Could you check a few things on this model? Use its own coordinates, in mm. Face numbers are marked on the shaded views. A direction names the side the tool comes from. Round coordinates to 2 decimals unless told otherwise and drop trailing zeros. Loops run counter-clockwise (first coordinate to the right, second up) from the corner with the lowest first, then second, coordinate; pieces in that order, holes last. Notation, with made-up numbers: (-35.75, 63) - (-25.75, 63) arc R20 ccw to (-25.75, 74) - close; hole circle Ø10 at (7.5, 15.25). An arc over 180 degrees is marked (long way). Use one line per item in the form item = value.
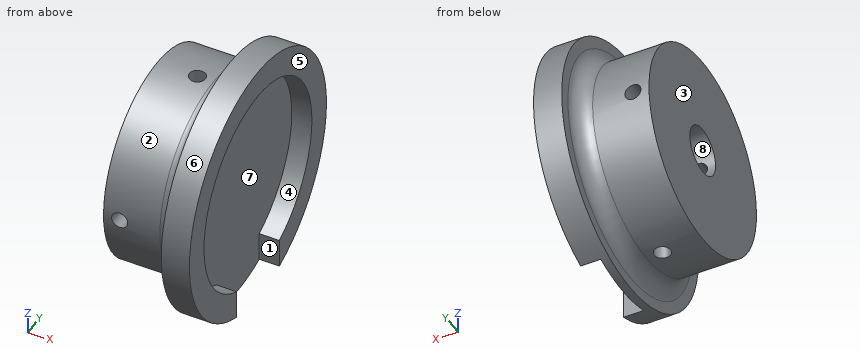
```python
from build123d import *

# Parameters (mm, degrees)
SKETCH_1_R                      = 12.55
EXTRUDE_1_DEPTH                 = 10
SKETCH_2_R                      = 3
CUT_EXTRUDE_1_DEPTH             = 7
CUT_EXTRUDE_2_REACH             = 22.372
SKETCH_3_R                      = 1
CUT_EXTRUDE_2_DIRECTION_2_REACH = 22.372
CUT_EXTRUDE_3_DEPTH             = 21
CUT_EXTRUDE_3_DEPTH_BACK        = 19
SKETCH_4_R                      = 1
EXTRUDE_2_DEPTH                 = 2.5
EXTRUDE_2_DEPTH_BACK            = 1
SKETCH_5_R                      = 16
SKETCH_6_R                      = 12.6
CUT_EXTRUDE_4_DEPTH             = 2.5
FILLET_1_R                      = 2
SKETCH_7_W                      = 2.5
SKETCH_7_H                      = 10
CUT_EXTRUDE_5_DEPTH             = 21.5


with BuildPart() as part:
    # 草图1 → 凸台-拉伸1 (new body)
    with BuildSketch(Plane(origin=(0, 0, 0), x_dir=(0, 0, -1), z_dir=(1, 0, 0))):
        Circle(SKETCH_1_R)
    extrude(amount=EXTRUDE_1_DEPTH)

    # 草图2 → 切除-拉伸1 (cut)
    with BuildSketch(Plane.ZY):
        Circle(SKETCH_2_R)
    extrude(amount=-CUT_EXTRUDE_1_DEPTH, mode=Mode.SUBTRACT)

    # 草图3 → 切除-拉伸2 (cut, up to next)
    with BuildSketch(Plane(origin=(0, 0, 0), x_dir=(1, 0, 0), z_dir=(0, 1, 0)), mode=Mode.PRIVATE) as cut_extrude_2_sk1:
        with Locations(Location((2, 0, 0), (0, 0, 270))):
            Circle(SKETCH_3_R)
    cut_extrude_2_tool1 = extrude(cut_extrude_2_sk1.sketch, amount=-CUT_EXTRUDE_2_REACH, mode=Mode.PRIVATE) & part.part
    add(cut_extrude_2_tool1.solids().sort_by_distance((2, 0, 0))[0], mode=Mode.SUBTRACT)

    # 草图3 → 切除-拉伸2 direction 2 (cut, up to next)
    with BuildSketch(Plane(origin=(0, 0, 0), x_dir=(1, 0, 0), z_dir=(0, 1, 0)), mode=Mode.PRIVATE) as cut_extrude_2_direction_2_sk1:
        with Locations(Location((2, 0, 0), (0, 0, 270))):
            Circle(SKETCH_3_R)
    cut_extrude_2_direction_2_tool1 = extrude(cut_extrude_2_direction_2_sk1.sketch, amount=CUT_EXTRUDE_2_DIRECTION_2_REACH, mode=Mode.PRIVATE) & part.part
    add(cut_extrude_2_direction_2_tool1.solids().sort_by_distance((2, 0, 0))[0], mode=Mode.SUBTRACT)

    # 草图4 → 切除-拉伸3 (cut, two sides: drawn at the far end of the back side and taken through both)
    with BuildSketch(Plane.XY.offset(-CUT_EXTRUDE_3_DEPTH_BACK)):
        with Locations(Location((5, 0, 0), (0, 0, 180))):
            Circle(SKETCH_4_R)
    extrude(amount=CUT_EXTRUDE_3_DEPTH + CUT_EXTRUDE_3_DEPTH_BACK, mode=Mode.SUBTRACT)

    # 草图5 → 凸台-拉伸2 (add, two sides: drawn at the far end of the back side and taken through both)
    with BuildSketch(Plane(origin=(10, 0, 0), x_dir=(0, 0, -1), z_dir=(1, 0, 0)).offset(-EXTRUDE_2_DEPTH_BACK)):
        Circle(SKETCH_5_R)
    extrude(amount=EXTRUDE_2_DEPTH + EXTRUDE_2_DEPTH_BACK)

    # 草图6 → 切除-拉伸4 (cut)
    with BuildSketch(Plane(origin=(12.5, 0, 0), x_dir=(0, 0, -1), z_dir=(1, 0, 0))):
        Circle(SKETCH_6_R)
    extrude(amount=-CUT_EXTRUDE_4_DEPTH, mode=Mode.SUBTRACT)

    # 圆角1
    fillet_1_edges = [part.edges().sort_by_distance(p)[0] for p in [
        (9, 0, 12.55),
    ]]
    fillet(fillet_1_edges, radius=FILLET_1_R)

    # 草图7 → 切除-拉伸5 (cut)
    with BuildSketch(Plane.XY):
        with Locations((11.25, 0)):
            Rectangle(SKETCH_7_W, SKETCH_7_H)
    extrude(amount=-CUT_EXTRUDE_5_DEPTH, mode=Mode.SUBTRACT)


solid = part.part
```
1. If we section it at C-C, the plane x = 5.5: Write out the boundary of the cut face in (y, z).
Solution:
outline = (-0.87, -12.52) - (-0.87, -2.87) arc R3 cw to (-0.87, 2.87) - (-0.87, 12.52) arc R12.55 ccw to start; (0.87, -12.52) arc R12.55 ccw to (0.87, 12.52) - (0.87, 2.87) arc R3 cw to (0.87, -2.87) - close
2. We'd pull the mould along Z, two halves only. Please class the marked faces 5, 6, 7 and 8: +Z half, -Z half, draft (parallel to the pull), parting line (faces both ways), or undercut.
Solution:
face_5 = draft
face_6 = parting line
face_7 = undercut
face_8 = undercut
3. For P1, Ø8, axis at y = 0, z = 0, coming from the +X side; P2, Ø1.5, axis at y = 3.5, z = -5, coming from the -X side; P3, Ø1.6, axis at x = 2, z = 0, coming from the -Y side; P4, Ø1, axis at x = 2.5, z = 6, coming from the -Y side, each with a flat end and sliding along its axis, tell me the tip position at first contact or that it passes through.
Solution:
P1 = 10
P2 = 0
P3 = through
P4 = -11.28
4. Please list where these lines run through material, in increasing order: line 1 along X through (y, z) = (6.5, -13); line 2 along Y through (x, z) = (4.25, 0); line 3 along Y through (x, z) = (4.75, -11.5).
Solution:
line_1 = 9 to 12.5
line_2 = -12.55 to -3, 3 to 12.55
line_3 = -5.03 to -0.97, 0.97 to 5.03
5. If we section it at D-D, the plane x = 9.5: Write out the boundary of the cut face in (y, z), plus the area to 3 significant figures.
Solution:
outline = circle Ø32 at (0, 0)
area = 804 mm^2
6. If we section it at B-B, the plane y = 0: Write out the boundary of the cut face in (x, z).
Solution:
outline = (0, -12.55) - (4, -12.55) - (4, -3) - (0, -3) - close; (0, 3) - (4, 3) - (4, 12.55) - (0, 12.55) - close; (6, -12.55) - (7, -12.55) arc R2 cw to (9, -14.55) - (9, -16) - (10, -16) - (10, 12.6) - (12.5, 12.6) - (12.5, 16) - (9, 16) - (9, 14.55) arc R2 cw to (7, 12.55) - (6, 12.55) - (6, 3) - (7, 3) - (7, -3) - (6, -3) - close
7. If we section it at A-A, the plane z = 0: Write out the boundary of the cut face in (x, y), plus the area to 3 significant figures.
Solution:
outline = (0, -12.55) - (1, -12.55) - (1, -3) - (0, -3) - close; (0, 3) - (1, 3) - (1, 12.55) - (0, 12.55) - close; (3, -12.55) - (7, -12.55) arc R2 cw to (9, -14.55) - (9, -16) - (12.5, -16) - (12.5, -12.6) - (10, -12.6) - (10, 12.6) - (12.5, 12.6) - (12.5, 16) - (9, 16) - (9, 14.55) arc R2 cw to (7, 12.55) - (3, 12.55) - (3, 3) - (7, 3) - (7, -3) - (3, -3) - close
area = 196 mm^2
8. On a 3-axis mill with a long thin cutter (end or side, diameter ignored), from which of +Z, -Z, +X, -X, +Y, -Y can I reach the whole of each face in a straight line? I mean the marked faces 1, 2, 3 and 4. Say none if no direction works.
Solution:
face_1 = -Z, +X
face_2 = -X
face_3 = +Z, -Z, -X, +Y, -Y
face_4 = +X
